```python
from build123d import *

# Parameters (mm, degrees)
BOSS_EXTRUDE1_DEPTH                             = 15
M5_CLEARANCE_HOLE1_D                            = 5.5
M5_CLEARANCE_HOLE2_D                            = 5.5
CBORE_FOR_M4_SOCKET_HEAD_CAP_SCREW1_D           = 4.5
CBORE_FOR_M4_SOCKET_HEAD_CAP_SCREW1_CBORE_D     = 8
CBORE_FOR_M4_SOCKET_HEAD_CAP_SCREW1_CBORE_DEPTH = 4
HOLE_WIZARD_M51_D                               = 4.2
HOLE_WIZARD_M51_DEPTH                           = 14
HOLE_WIZARD_M51_TIP                             = 1.2618073


with BuildPart() as part:
    # Sketch1 → Boss-Extrude1 (new body)
    with BuildSketch(Plane(origin=(0, 0, 0), x_dir=(1, 0, 0), z_dir=(0, 1, 0))):
        Polygon((0, 100), (30, 130), (137, 130), (137, 120), (137, 45), (87, 0), (5, 0), (0, 5), align=None)
    extrude(amount=BOSS_EXTRUDE1_DEPTH)

    # M5 Clearance Hole1 (through all)
    with Locations(Plane(origin=(0, 15, 0), x_dir=(-1, 0, 0), z_dir=(0, 1, 0))):
        with Locations((-100, -59.5), (-100, -113.5)):
            Hole(M5_CLEARANCE_HOLE1_D / 2)

    # M5 Clearance Hole2 (through all)
    with Locations(Plane(origin=(0, 15, 0), x_dir=(-1, 0, 0), z_dir=(0, 1, 0))):
        with Locations((-131, -111.5), (-131, -61.5)):
            Hole(M5_CLEARANCE_HOLE2_D / 2)

    # CBORE for M4 Socket Head Cap Screw1 (through all)
    with Locations(Plane(origin=(0, 15, 0), x_dir=(-1, 0, 0), z_dir=(0, 1, 0))):
        with Locations((-12.5, -91.5), (-12.5, -57.5), (-54.5, -57.5), (-54.5, -91.5)):
            CounterBoreHole(CBORE_FOR_M4_SOCKET_HEAD_CAP_SCREW1_D / 2, CBORE_FOR_M4_SOCKET_HEAD_CAP_SCREW1_CBORE_D / 2, CBORE_FOR_M4_SOCKET_HEAD_CAP_SCREW1_CBORE_DEPTH)

    # Отверстие обработанное метчиком M51
    with Locations(Plane.ZY):
        with Locations((-50, 7.5), (-20, 7.5)):
            Hole(HOLE_WIZARD_M51_D / 2, depth=HOLE_WIZARD_M51_DEPTH)
            with Locations((0, 0, -(HOLE_WIZARD_M51_DEPTH + HOLE_WIZARD_M51_TIP / 2))):  # 118° drill point
                Cone(0, HOLE_WIZARD_M51_D / 2, HOLE_WIZARD_M51_TIP, mode=Mode.SUBTRACT)


solid = part.part
```
The model under review builds one solid part; all positions refer to its coordinate system, in mm. A direction names the side the tool comes from. Round coordinates to 2 decimals unless told otherwise and drop trailing zeros. Loops run counter-clockwise (first coordinate to the right, second up) from the corner with the lowest first, then second, coordinate; pieces in that order, holes last. Notation, with made-up numbers: M -38.75,-13 L -1.75,-13 A17 cw -1.75,-9 Z; hole C -4,88.25 d8. An arc over 180 degrees is marked long. Answer as a JSON object with one key per item and string values.
(1) To check wall thickness, follow line 1 along Z through (x, y) = (54.5, 2.5); line 2 along Z through (x, y) = (54.5, 14); line 3 along X through (y, z) = (3.5, -64). State the ranges of each line that lie inside material, in increasing order.
Resolved:
{"line 1": "-130 to -93.75, -89.25 to -59.75, -55.25 to 0", "line 2": "-130 to -95.5, -87.5 to -61.5, -53.5 to 0", "line 3": "0 to 129.85, 132.15 to 137"}
(2) Clearance check with flat-ended pins moving along their axes: P1, Ø4, axis at x = 55.5, z = -93.5, coming from the +Y side; P2, Ø3.5, axis at x = 131, z = -61.5, coming from the +Y side; P3, Ø6, axis at x = 26.5, y = 2, coming from the -Z side. State where each tip first meets the part, or that it passes through.
Resolved:
{"P1": "y = 15", "P2": "through", "P3": "z = -129.5"}
(3) Tool access review of faces 5 (the cylindrical face through (132.27, 7.4, -113.94)), 6 (the flat face through (10.8, 11, -93.2)): name each direction out of +Z, -Z, +X, -X, +Y, -Y from which nothing blocks a thin tool from reaching the whole face with its end or side.
Resolved:
{"face 5": "+Y, -Y", "face 6": "+Y"}
(4) Take a section at C-C on z = -121.5. Give the boundary of the cut face in (x, y).
Resolved:
{"outline": "M 21.5,0 L 137,0 L 137,15 L 21.5,15 Z"}
(5) Draft analysis for pull direction Z (two halves, no side actions). For faces 1 (the flat face through (47, 7, 0)), 2 (the flat face through (15, 7, -115)), 3 (the cylindrical face through (13.367, 13.028, -95.405)), 4 (the flat face through (69, 15, -66)), state which applies: released by +Z, released by -Z, zero draft, split by the parting line, or undercut.
Resolved:
{"face 1": "released by +Z", "face 2": "released by -Z", "face 3": "undercut", "face 4": "zero draft"}
(6) Take a section at A-A on x = 100. Give the boundary of the cut face in (y, z), and give its area (3 significant figures).
Resolved:
{"outline": "M 0,-130 L 15,-130 L 15,-116.25 L 0,-116.25 Z; M 0,-110.75 L 15,-110.75 L 15,-62.25 L 0,-62.25 Z; M 0,-56.75 L 15,-56.75 L 15,-11.7 L 0,-11.7 Z", "area": "1,610 mm²"}
(7) Take a section at B-B on y = 2. Count the separate pieces of the cut face and the enclosed holes in it, and give its area (3 significant figures).
Resolved:
{"separate pieces": "1", "enclosed holes": "8", "area": "16,100 mm²"}
